The drawing under review shows one solid part. Ordinate dimensions are in mm from its lowest x, y, z. A direction names the side the tool comes from. Round coordinates to 2 decimals unless told otherwise and drop trailing zeros. Order: outer loops, then holes, each group sorted by start corner. A loop starts at its lowest first (then second) coordinate and runs counter-clockwise, first axis right, second up.
1) To check wall thickness, follow L1, parallel to Z at x = 70, y = 14.5; L2, parallel to Z at x = 70, y = 29; L3, parallel to X at y = 20, z = 56.5. State the ranges of each line that lie inside material, in increasing order.
2) Consider section B-B (x = 86.5). Give the boundary of the cut face in (y, z), then the cut area to 3 significant figures.
3) Consider section D-D (x = 17). Give the boundary of the cut face in (y, z).
4) Machinability: for the marked faces 5 and 6, which of the approach directions +Z, -Z, +X, -X, +Y, -Y give a long, thin tool a straight path to every point of the face, cutting with its end or side? Answer none if there is none.
5) Mouldability with a two-part tool opening along Z and no side actions: class the marked faces 1, 2, 3 and 4 as pulls with the +Z half, pulls with the -Z half, needs draft (parallel to the pull), parting line crosses it, or undercut.
6) Consider section C-C (y = 49). Give the boundary of the cut face in (x, z), then the cut area to 3 significant figures.
7) Clearance check with flat-ended pins moving along their axes: P1, Ø6, axis at y = 23, z = 66, coming from the +X side; P2, Ø1.5, axis at x = 84, y = 42, coming from the -Z side; P3, Ø4, axis at y = 40.5, z = 62, coming from the +X side. State where each tip first meets the part, or that it passes through.
8) Consider section A-A (z = 70). Give the boundary of the cut face in (x, y).
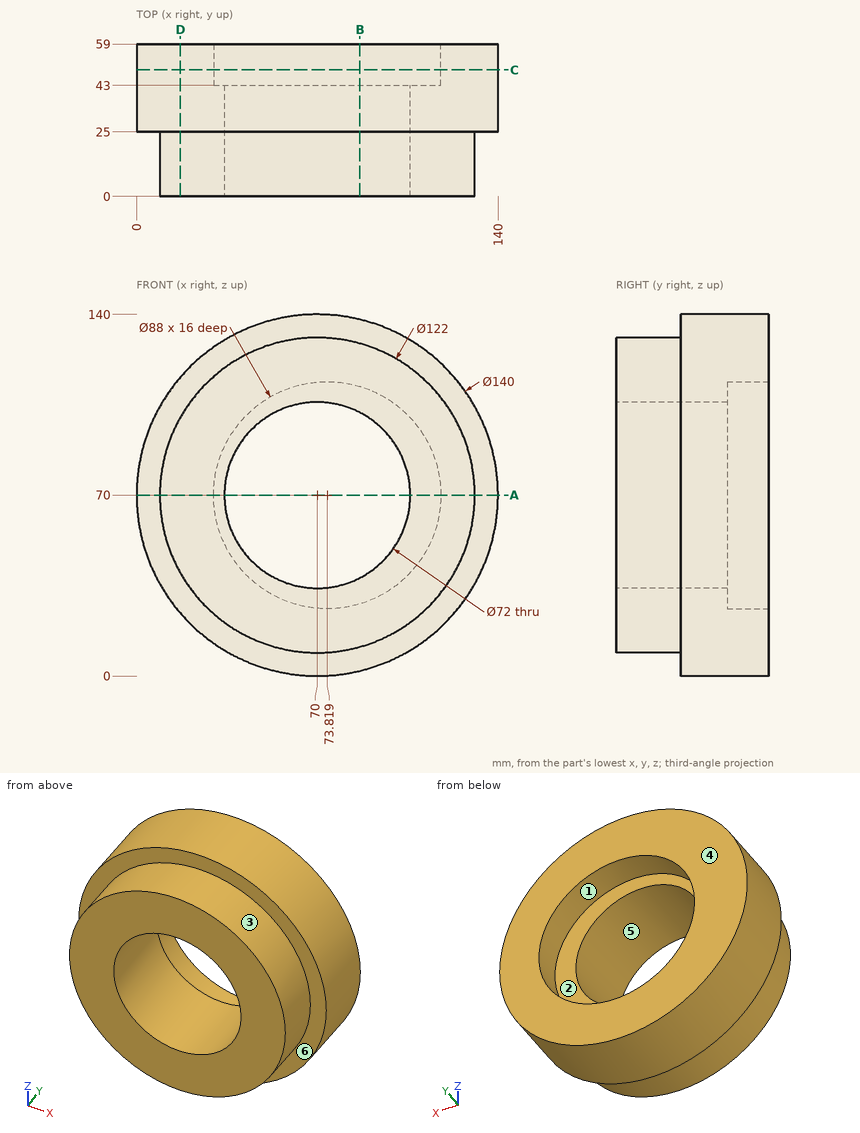
Answer below:
1. L1: z = 9 to 34, 106 to 131
1. L2: z = 0 to 34, 106 to 140
1. L3: x = 10.51 to 36.63, 103.37 to 129.49
2. outline: (0, 11.27) - (25, 11.27) - (25, 1.97) - (59, 1.97) - (59, 27.87) - (43, 27.87) - (43, 38) - (0, 38) - close; (0, 102) - (43, 102) - (43, 112.13) - (59, 112.13) - (59, 138.03) - (25, 138.03) - (25, 128.73) - (0, 128.73) - close
2. area: 3,460 mm2
3. outline: (0, 39.8) - (25, 39.8) - (25, 24.27) - (59, 24.27) - (59, 115.73) - (25, 115.73) - (25, 100.2) - (0, 100.2) - close
4. face 5: +Y, -Y
4. face 6: -Y
5. face 1: undercut
5. face 2: undercut
5. face 3: parting line crosses it
5. face 4: needs draft
6. outline: circle Ø140 at (70, 70); hole circle Ø88 at (73.82, 70)
6. area: 9,310 mm2
7. P1: stops at x = 139.98
7. P2: stops at z = 1.27
7. P3: stops at x = 139.74
8. outline: (0, 25) - (9, 25) - (9, 0) - (34, 0) - (34, 43) - (29.82, 43) - (29.82, 59) - (0, 59) - close; (106, 0) - (131, 0) - (131, 25) - (140, 25) - (140, 59) - (117.82, 59) - (117.82, 43) - (106, 43) - close
